```python
from build123d import *

# Parameters (mm, degrees)
SKETCH_1_R          = 5.75
EXTRUDE_1_DEPTH     = 1
SKETCH_1_R_2        = 25
SKETCH_1_R_3        = 1.5
SKETCH_1_R_4        = 5.5
EXTRUDE_1_2_DEPTH   = 1
EXTRUDE_2_DEPTH     = 1
SKETCH_3_R          = 5.75
EXTRUDE_3_DEPTH     = 30
CUT_EXTRUDE_1_DEPTH = 30
EXTRUDE_4_DEPTH     = 2
SKETCH_6_R          = 4.75
CUT_EXTRUDE_3_DEPTH = 30


with BuildPart() as part:
    # Sketch 1 → Extrude 1 (new body)
    with BuildSketch(Plane(origin=(0, 0, 0), x_dir=(1, 0, 0), z_dir=(0, 1, 0))):
        with Locations((37.5, -42.927264064)):
            Circle(SKETCH_1_R)
    extrude(amount=EXTRUDE_1_DEPTH)



with BuildPart() as body_2:
    # Sketch 1 → Extrude 1 2 (new body)
    with BuildSketch(Plane(origin=(0, 0, 0), x_dir=(1, 0, 0), z_dir=(0, 1, 0))):
        Circle(SKETCH_1_R_2)
        with Locations((0, -18)):
            Circle(SKETCH_1_R_3, mode=Mode.SUBTRACT)
        with Locations((-12.727922061, -12.727922061)):
            Circle(SKETCH_1_R_3, mode=Mode.SUBTRACT)
        with Locations((-18, 0)):
            Circle(SKETCH_1_R_3, mode=Mode.SUBTRACT)
        with Locations((-12.727922061, 12.727922061)):
            Circle(SKETCH_1_R_3, mode=Mode.SUBTRACT)
        with Locations((0, 18)):
            Circle(SKETCH_1_R_3, mode=Mode.SUBTRACT)
        with Locations((12.727922061, 12.727922061)):
            Circle(SKETCH_1_R_3, mode=Mode.SUBTRACT)
        with Locations((18, 0)):
            Circle(SKETCH_1_R_3, mode=Mode.SUBTRACT)
        with Locations((12.727922061, -12.727922061)):
            Circle(SKETCH_1_R_3, mode=Mode.SUBTRACT)
        Circle(SKETCH_1_R_4, mode=Mode.SUBTRACT)
    extrude(amount=EXTRUDE_1_2_DEPTH)


with BuildPart() as part_1:
    add(part.part)

    add(body_2.part)  # Extrude 2 merges body 2
    # Sketch 2 → Extrude 2 (add)
    with BuildSketch(Plane(origin=(0, 0, 0), x_dir=(1, 0, 0), z_dir=(0, 1, 0))):
        with BuildLine():
            Line((0, -25), (33.976022053, -47.470839685))
            ThreePointArc((33.976022053, -47.470839685), (37.308300147, -42.73151924), (42.116158776, -39.498914876))
            Line((42.116158776, -39.498914876), (25, 0))
            Line((25, 0), (15.739254024, -17.717074967))
            Line((15.739254024, -17.717074967), (0, -25))
        make_face()
    extrude(amount=EXTRUDE_2_DEPTH)

    # Sketch 3 → Extrude 3 (add)
    with BuildSketch(Plane(origin=(0, 0, 0), x_dir=(1, 0, 0), z_dir=(0, 1, 0))):
        with Locations((37.5, -42.927264064)):
            Circle(SKETCH_3_R)
    extrude(amount=EXTRUDE_3_DEPTH)

    # Sketch 4 → Cut-Extrude 1 (cut)
    with BuildSketch(Plane(origin=(0, 1, 0), x_dir=(1, 0, 0), z_dir=(0, 1, 0))):
        Polygon((16.101209637, -18.431490076), (22.006815823, -13.272525562), (33.717105263, -38.596882163), (10.14517855, -23.634504306), align=None)
    extrude(amount=-CUT_EXTRUDE_1_DEPTH, mode=Mode.SUBTRACT)

    # Sketch 5 → Extrude 4 (add)
    with BuildSketch(Plane(origin=(0, 1, 0), x_dir=(1, 0, 0), z_dir=(0, 1, 0))):
        Polygon((31.75, -42.927264064), (4.342000799, -24.620053393), (7.010063543, -23.99706251), (32.159659881, -40.79576989), align=None)
        Polygon((38.971739634, -37.368803625), (24.515251473, -4.899229044), (23.694530655, -7.973030605), (36.720800315, -37.230304537), align=None)
    extrude(amount=EXTRUDE_4_DEPTH)

    # Sketch 6 → Cut-Extrude 3 (cut)
    with BuildSketch(Plane(origin=(0, 30, 0), x_dir=(1, 0, 0), z_dir=(0, 1, 0))):
        with Locations((37.5, -42.927264064)):
            Circle(SKETCH_6_R)
    extrude(amount=-CUT_EXTRUDE_3_DEPTH, mode=Mode.SUBTRACT)


solid = part_1.part
```
Input: part model. Units: mm. Frame: model coordinates. A direction names the side the tool comes from. Coordinates: 2 decimals unless noted, no trailing zeros. Loops run counter-clockwise (first coordinate to the right, second up) from the corner with the lowest first, then second, coordinate; pieces in that order, holes last. Notation, with made-up numbers: M 27,-7 L 63,-7 A22 ccw 63,17 Z; hole C 85,-12.5 d11. An arc over 180 degrees is marked long. Use a Markdown table: item, result. Add a question column.
1) Pin query (flat end, axial travel): P1, Ø2.5, axis at x = -18, z = 0, coming from the +Y side; P2, Ø4, axis at x = 12.73, z = -12.73, coming from the -Y side; P3, Ø12, axis at x = 29, y = 12.5, coming from the +Z side; P4, Ø8, axis at x = 1, z = -10.5, coming from the +Y side. Return the tip coordinate at first contact, or that it passes through.
2) Section D-D, the plane x = 35.5. Return the cut outline in (y, z).
3) Set-up query: faces 1 (the flat face through (31.845, 1.986, 21.361)), 2 (the flat face through (38, 30, 38)), 3 (the cylindrical face through (14.11, 0.49, -12.15)), 4 (the flat face through (18.238, 1.986, 33.902)), 5 (the flat face through (5.657, 1.986, 24.313)). Return all of +Z, -Z, +X, -X, +Y, -Y with unobstructed straight access to the full face (end or side cutting, diameter ignored); none if empty.
4) Section A-A, the plane x = 18. Return the cut outline in (y, z).
5) Line query: L1, parallel to Z at x = 0, y = 0.2; L2, parallel to Z at x = 37.5, y = 12.25. Output: solid intervals per line, ascending. Write a range as from..to.
6) Section C-C, the plane y = 4. Return the cut outline in (x, z), plus the area to 3 significant figures.
7) Section B-B, the plane z = 26. Return the cut outline in (x, y), plus the area to 3 significant figures.
8) Draft query along Z for faces 6 (the flat face through (27.8, 0.5, 25.8)), 7 (the flat face through (24.11, 1.99, 6.41)), 8 (the flat face through (19.41, 1.99, 32.28)), 9 (the cylindrical face through (-17.085, 0.493, -18.251)). Return one class per face: +Z half, -Z half, draft (parallel to the pull), parting line (faces both ways), or undercut.
Answer below:
| question | item | result |
|---|---|---|
| 1 | P1 | through |
| 1 | P2 | y = 0 |
| 1 | P3 | z = 48.11 |
| 1 | P4 | y = 1 |
| 2 | outline | M 0,24.23 L 1,24.23 L 1,29.57 L 3,29.57 L 3,34.49 L 1,34.49 L 1,37.54 L 30,37.54 L 30,38.62 L 0,38.62 Z; M 0,47.24 L 30,47.24 L 30,48.32 L 0,48.32 Z |
| 3 | face 1 | -Z, +X, +Y |
| 3 | face 2 | +Z, -Z, +X, -X, +Y |
| 3 | face 3 | +Y, -Y |
| 3 | face 4 | +Z, -X, +Y |
| 3 | face 5 | -Z, -X, +Y |
| 4 | outline | M 0,-17.35 L 1,-17.35 L 1,-1.5 L 0,-1.5 Z; M 0,1.5 L 1,1.5 L 1,16.77 L 0,16.77 Z; M 0,28.62 L 1,28.62 L 1,31.34 L 3,31.34 L 3,33.74 L 1,33.74 L 1,36.9 L 0,36.9 Z |
| 5 | L1 | -25..-19.5, -16.5..-5.5, 5.5..16.5, 19.5..25 |
| 5 | L2 | 37.18..38.18, 47.68..48.68 |
| 6 | outline | C 37.5,42.93 d11.5; hole C 37.5,42.93 d9.5 |
| 6 | area | 33.0 mm2 |
| 7 | outline | M 1.51,0 L 13.87,0 L 13.87,1 L 10.01,1 L 10.01,3 L 6.41,3 L 6.41,1 L 1.51,1 Z; M 27.89,0 L 36.27,0 L 36.27,1 L 33.91,1 L 33.91,3 L 31.72,3 L 31.72,1 L 27.89,1 Z |
| 7 | area | 32.3 mm2 |
| 8 | face 6 | undercut |
| 8 | face 7 | -Z half |
| 8 | face 8 | undercut |
| 8 | face 9 | parting line |
